Geometry check sheet. Reference: the model listing, model coordinates, mm. Face numbers are marked on the shaded views. Round coordinates to 2 decimals unless told otherwise and drop trailing zeros. Write each loop counter-clockwise with the first axis right and the second up, starting at its lowest first coordinate (ties: lowest second). Pieces come first, ordered by that corner, then holes.
from build123d import *

# Parameters (mm, degrees)
SKETCH1_R           = 12.5
SKETCH1_R_2         = 1.190625
SKETCH1_R_3         = 3.3782
BOSS_EXTRUDE1_DEPTH = 40
SKETCH2_W           = 7.5
SKETCH2_H           = 24
SKETCH2_W_2         = 2.4
SKETCH2_H_2         = 5.75


with BuildPart() as part:
    # Sketch1 → Boss-Extrude1 (new body)
    with BuildSketch(Plane(origin=(0, 0, 0), x_dir=(0, 1, 0), z_dir=(0, 0, 1))):
        with Locations(Location((0, 0, 0), (0, 0, 270))):
            Circle(SKETCH1_R)
        with Locations(Location((0, -7.5, 0), (0, 0, 270))):
            Circle(SKETCH1_R_2, mode=Mode.SUBTRACT)
        with Locations(Location((7.5, 0, 0), (0, 0, 270))):
            Circle(SKETCH1_R_2, mode=Mode.SUBTRACT)
        with Locations(Location((-7.5, 0, 0), (0, 0, 270))):
            Circle(SKETCH1_R_2, mode=Mode.SUBTRACT)
        with Locations(Location((0, 7.5, 0), (0, 0, 270))):
            Circle(SKETCH1_R_2, mode=Mode.SUBTRACT)
        with Locations(Location((0, 0, 0), (0, 0, 270))):
            Circle(SKETCH1_R_3, mode=Mode.SUBTRACT)
    extrude(amount=BOSS_EXTRUDE1_DEPTH)

    # Sketch2 → Revolve1 (revolve)
    with BuildSketch(Plane.YZ, mode=Mode.PRIVATE) as revolve1_sk:
        with Locations((-8.75, 20)):
            Rectangle(SKETCH2_W, SKETCH2_H)
        with Locations((-13.7, 37.125)):
            Rectangle(SKETCH2_W_2, SKETCH2_H_2)
    revolve(revolve1_sk.sketch.rotate(Axis((0, 0, 0), (0, 0, 1)), 270), axis=Axis((0, 0, 0), (0, 0, 1)))


solid = part.part
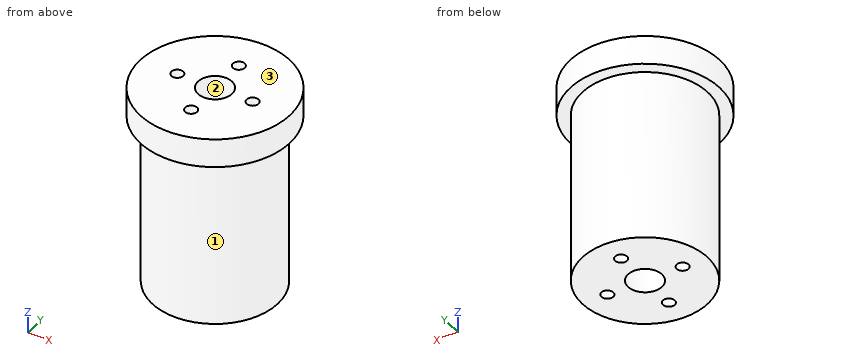
1. Section check C-C (x = -2.5). Record the cut outline in (y, z), plus the area to 3 significant figures.
2. Depth check by flat-ended pin: pin 1 Ø0.7 at (x, y) = (-0.5, -7.5) entering from +Z; pin 2 Ø0.7 at (x, y) = (-8, -0.5) entering from -Z; pin 3 Ø8 at (x, z) = (-1.5, 17) entering from -Y; pin 4 Ø2 at (x, y) = (5.5, -3) entering from -Z. Enter the tip coordinate at first touch or a pass-through.
3. Section check D-D (z = 10). Record the cut outline in (x, y).
4. Release check for a two-part mould opening along Y. For the marked faces 1, 2 and 3 record: +Y half, -Y half, draft (parallel to the pull), parting line (faces both ways), or undercut.
5. Section check A-A (y = 0). Record the cut outline in (x, z).
6. Section check B-B (z = 37). Record the cut outline in (x, y).
7. Scan lines: line 1 along Y through (x, z) = (0, 35.5); line 2 along Y through (x, z) = (0, 20); line 3 along X through (y, z) = (-0.5, 7). Record each from-to range of solid material in increasing order.
Results below:
1. outline: (-14.69, 34.25) - (-12.25, 34.25) - (-12.25, 0) - (-2.27, 0) - (-2.27, 40) - (-14.69, 40) - close; (2.27, 0) - (12.25, 0) - (12.25, 34.25) - (14.69, 34.25) - (14.69, 40) - (2.27, 40) - close
1. area: 826 mm2
2. pin 1: stops at z = 32
2. pin 2: stops at z = 8
2. pin 3: stops at y = -12.5
2. pin 4: stops at z = 0
3. outline: circle Ø25 at (0, 0); hole circle Ø6.76 at (0, 0)
4. face 1: parting line
4. face 2: undercut
4. face 3: draft
5. outline: (-14.9, 34.25) - (-12.5, 34.25) - (-12.5, 0) - (-8.69, 0) - (-8.69, 8) - (-6.31, 8) - (-6.31, 0) - (-3.38, 0) - (-3.38, 40) - (-6.31, 40) - (-6.31, 32) - (-8.69, 32) - (-8.69, 40) - (-14.9, 40) - close; (3.38, 0) - (6.31, 0) - (6.31, 8) - (8.69, 8) - (8.69, 0) - (12.5, 0) - (12.5, 34.25) - (14.9, 34.25) - (14.9, 40) - (8.69, 40) - (8.69, 32) - (6.31, 32) - (6.31, 40) - (3.38, 40) - close
6. outline: circle Ø29.8 at (0, 0); hole circle Ø2.38 at (-7.5, 0); hole circle Ø6.76 at (0, 0); hole circle Ø2.38 at (0, -7.5); hole circle Ø2.38 at (0, 7.5); hole circle Ø2.38 at (7.5, 0)
7. line 1: y = -14.9 to -8.69, -6.31 to -3.38, 3.38 to 6.31, 8.69 to 14.9
7. line 2: y = -12.5 to -3.38, 3.38 to 12.5
7. line 3: x = -12.49 to -8.58, -6.42 to -3.34, 3.34 to 6.42, 8.58 to 12.49
